Build history of the part. All positions in model axes, mm. A direction names the side the tool comes from. Give positions to 0.01 mm unless a question says otherwise; leave off trailing zeros. Loops run counter-clockwise (first coordinate to the right, second up) from the corner with the lowest first, then second, coordinate; pieces in that order, holes last. Notation, with made-up numbers: (-14.75, 64.5) -> (-3.75, 64.5) arc R17 ccw to (-3.75, 87.5) -> close; hole circle Ø2 at (-5, 62). An arc over 180 degrees is marked (long way). One line per question, with ' | ' between items. Start each with the question number.
(1) Slice it at A-A, the plane x = 0. Write the cut outline in (y, z), then the cut area to 3 significant figures.
(2) Slice it at D-D, the plane z = 4.05. Write the cut outline in (x, y).
(3) 3-axis set-ups, long thin cutter, end or side, ignore diameter. For faces 1 (the face through (0.867, 3.905, 1.312)), 2 (the face through (0, 0, 0)): which of +Z, -Z, +X, -X, +Y, -Y reach the whole face in a straight line?
(4) Drill centre lines: L1, parallel to Z at x = 7, y = 0.25; L2, parallel to Y at x = 0, z = 4.9; L3, parallel to Z at x = -1.5, y = 3.75. Where is each one in solid material? Low to high. Write a range as from..to.
(5) Flat gauge pin, fed straight in: pin 1 Ø2 at (y, z) = (2, 3.5) entering from +X. Where does the tip first touch, or does it go through?
(6) Slice it at C-C, the plane z = 1.7. Write the cut outline in (x, y).
```python
from build123d import *

# Parameters (mm, degrees)
F2_R     = 0.5
F3_SIZE2 = 0.2
F3_SIZE  = 0.4


with BuildPart() as f1:
    # F0 (on Front) → F1 (revolve)
    with BuildSketch(Plane.XZ):
        Polygon((-4, 0), (0, 0), (0, 5.25), (-9, 5.25), (-9, 3.25), (-5.25, 3.25), (-5.25, 2.25), (-4, 2.25), align=None)
    revolve(axis=Axis((0, 0, 2.625), (0, 0, 1)))

    # F2
    f2_edges = [f1.edges().sort_by_distance(p)[0] for p in [
        (9, 0, 3.25),
    ]]
    fillet(f2_edges, radius=F2_R)

    # F3
    f3_edges = [f1.edges().sort_by_distance(p)[0] for p in [
        (4, 0, 0),
    ]]
    f3_side = f1.faces().sort_by_distance((4, 0, 1.125))[0]
    chamfer(f3_edges, length=F3_SIZE, length2=F3_SIZE2, reference=f3_side)


solid = f1.part
```
Final values:
1) outline: (-9, 3.75) arc R0.5 ccw to (-8.5, 3.25) -> (-5.25, 3.25) -> (-5.25, 2.25) -> (-4, 2.25) -> (-4, 0.4) -> (-3.8, 0) -> (3.8, 0) -> (4, 0.4) -> (4, 2.25) -> (5.25, 2.25) -> (5.25, 3.25) -> (8.5, 3.25) arc R0.5 ccw to (9, 3.75) -> (9, 5.25) -> (-9, 5.25) -> close | area: 64.3 mm2
2) outline: circle Ø18 at (0, 0)
3) face 1: -Z | face 2: -Z, +X, -X, +Y, -Y
4) L1: 3.25..5.25 | L2: -9..9 | L3: 2.25..5.25
5) pin 1: x = 8.94
6) outline: circle Ø8 at (0, 0)
